from build123d import *

# Parameters (mm, degrees)
ESQUISSE1_W             = 25
ESQUISSE1_H             = 25
BOSS_EXTRU_1_DEPTH      = 5
ESQUISSE3_R             = 1.45
ESQUISSE3_W             = 5
ESQUISSE3_H             = 5
ENL_V_MAT_EXTRU_1_DEPTH = 5
ESQUISSE5_R             = 2
ENL_V_MAT_EXTRU_2_DEPTH = 10


with BuildPart() as part:
    # Esquisse1 → Boss.-Extru.1 (new body)
    with BuildSketch(Plane.XY):
        with Locations((-53.521610088, -25.407575758)):
            Rectangle(ESQUISSE1_W, ESQUISSE1_H)
    boss_extru_1 = extrude(amount=BOSS_EXTRU_1_DEPTH)

    # Esquisse3 → Enlèv. mat.-Extru.1 (cut)
    with BuildSketch(Plane(origin=(0, 0, 0), x_dir=(-1, 0, 0), z_dir=(0, 0, -1))):
        with Locations((49.721610088, -29.457575758)):
            Circle(ESQUISSE3_R)
        Polygon((46.021610088, -22.907575758), (46.021610088, -17.907575758), (51.021610088, -17.907575758), (51.021610088, -12.907575758), (41.021610088, -12.907575758), (41.021610088, -22.907575758), align=None)
        with Locations((43.521610088, -30.407575758)):
            Rectangle(ESQUISSE3_W, ESQUISSE3_H)
        with Locations((58.521610088, -15.407575758)):
            Rectangle(ESQUISSE3_W, ESQUISSE3_H)
    enl_v_mat_extru_1 = extrude(amount=-ENL_V_MAT_EXTRU_1_DEPTH, mode=Mode.SUBTRACT)

    # Symétrie1: Boss.-Extru.1, Enlèv. mat.-Extru.1 across plane
    add(boss_extru_1.mirror(Plane(origin=(-66.021610088, -12.907575758, 5), x_dir=(0, 0, 1), z_dir=(1, 0, 0))))
    add(enl_v_mat_extru_1.mirror(Plane(origin=(-66.021610088, -12.907575758, 5), x_dir=(0, 0, 1), z_dir=(1, 0, 0))), mode=Mode.SUBTRACT)

    # Esquisse5 → Enlèv. mat.-Extru.2 (cut)
    with BuildSketch(Plane.XY.offset(5)):
        with Locations((-66.021610088, -28.907575758)):
            Circle(ESQUISSE5_R)
    extrude(amount=-ENL_V_MAT_EXTRU_2_DEPTH, mode=Mode.SUBTRACT)


solid = part.part
CAD build for the part. Positions are in the model's coordinates, mm. A direction names the side the tool comes from. Coordinates: 2 decimals unless noted, no trailing zeros. Order: outer loops, then holes, each group sorted by start corner. A loop starts at its lowest first (then second) coordinate and runs counter-clockwise, first axis right, second up.
Item 1: Band-saw the part on B-B on y = -16. List the corners of the cut face in (x, z), plus the area to 3 significant figures.
Check sheet entries:
outline: (-81.02, 0) - (-76.02, 0) - (-76.02, 5) - (-81.02, 5) - close; (-71.02, 0) - (-61.02, 0) - (-61.02, 5) - (-71.02, 5) - close; (-56.02, 0) - (-51.02, 0) - (-51.02, 5) - (-56.02, 5) - close
area: 100 mm2
Item 2: Band-saw the part on A-A on x = -50.5. List the corners of the cut face in (y, z).
Check sheet entries:
outline: (-37.91, 0) - (-30.68, 0) - (-30.68, 5) - (-37.91, 5) - close; (-28.23, 0) - (-17.91, 0) - (-17.91, 5) - (-28.23, 5) - close
Item 3: Band-saw the part on C-C on z = 0.6. Give the number of separate pieces and of enclosed holes in the cut face, plus the area to 3 significant figures.
Check sheet entries:
separate pieces: 1
enclosed holes: 3
area: 974 mm2
Item 4: Drill centre lines: L1, parallel to X at y = -14.75, z = 1.05; L2, parallel to X at y = -29, z = 2.7; L3, parallel to X at y = -32.5, z = 0.95. Where is each one in solid material? Low to high.
Check sheet entries:
L1: x = -81.02 to -76.02, -71.02 to -61.02, -56.02 to -51.02
L2: x = -86.02 to -83.7, -80.95 to -68.02, -64.02 to -51.1, -48.35 to -46.02
L3: x = -86.02 to -46.02
Item 5: 3-axis set-ups, long thin cutter, end or side, ignore diameter. For faces 4 (the face through (-71.022, -15, 2)), 5 (the face through (-84, -17.908, 2)), 6 (the face through (-51.022, -15, 2)), 7 (the face through (-89, -32.908, 2)): which of +Z, -Z, +X, -X, +Y, -Y reach the whole face in a straight line?
Check sheet entries:
face 4: +Z, -Z, +Y
face 5: +Z, -Z, -X, +Y
face 6: +Z, -Z, +X, +Y
face 7: +Z, -Z, -X
Item 6: Pin check, flat tips, straight feed: pin 1 Ø2.5 at (x, z) = (-59.5, 3.5) entering from +Y; pin 2 Ø2.5 at (y, z) = (-16.5, 2) entering from +X; pin 3 Ø1 at (y, z) = (-30.5, 3.5) entering from +X. Stop position of each tip, or through.
Check sheet entries:
pin 1: stops at y = -17.91
pin 2: stops at x = -51.02
pin 3: stops at x = -46.02
Item 7: Two-plate mould, pull along Y, no slides. Class faces 1 (the face through (-78, -12.908, 2)), 2 (the face through (-46.022, -30, 2)), 3 (the face through (-91.022, -35, 2)): +Y half, -Y half, draft (parallel to the pull), parting line (faces both ways), or undercut.
Check sheet entries:
face 1: +Y half
face 2: undercut
face 3: draft
Item 8: Band-saw the part on D-D on x = -66.5. List the corners of the cut face in (y, z), plus the area to 3 significant figures.
Check sheet entries:
outline: (-37.91, 0) - (-30.85, 0) - (-30.85, 5) - (-37.91, 5) - close; (-26.97, 0) - (-12.91, 0) - (-12.91, 5) - (-26.97, 5) - close
area: 106 mm2
